Can you work these out from the model? Positions are in its coordinate system, mm. Face numbers are marked on the shaded views. A direction names the side the tool comes from. Round coordinates to 2 decimals unless told otherwise and drop trailing zeros. Loops run counter-clockwise (first coordinate to the right, second up) from the corner with the lowest first, then second, coordinate; pieces in that order, holes last. Notation, with made-up numbers: M 37.5,45.25 L 68.5,45.25 A29 ccw 68.5,80.25 Z; hole C 52,84.25 d1. An arc over 180 degrees is marked long. Return JSON: item names as keys, results as strings.
```python
from build123d import *

# Parameters (mm, degrees)
SM_BASE_FLANGE_2_DEPTH = 28
SKETCH_10_R            = 1.45
SKETCH_10_R_2          = 1.7
CUT_EXTRUDE_1_DEPTH    = 73.725511342
SKETCH_12_R            = 1.6
SKETCH_12_R_2          = 1.7
CUT_EXTRUDE_3_DEPTH    = 4


# Sheet-metal steps are written as plain solids
with BuildPart() as part:
    # 草图1 → 基体-法兰2 (new body)
    with BuildSketch(Plane.XY):
        with BuildLine():
            Line((-27.5, -25), (-27.5, 23))
            ThreePointArc((-27.5, 23), (-26.914213562, 24.414213562), (-25.5, 25))
            Line((-25.5, 25), (25.5, 25))
            ThreePointArc((25.5, 25), (26.914213562, 24.414213562), (27.5, 23))
            Line((27.5, 23), (27.5, -25))
            Line((27.5, -25), (30.5, -25))
            Line((30.5, -25), (30.5, 23))
            ThreePointArc((30.5, 23), (29.035533906, 26.535533906), (25.5, 28))
            Line((25.5, 28), (-25.5, 28))
            ThreePointArc((-25.5, 28), (-29.035533906, 26.535533906), (-30.5, 23))
            Line((-30.5, 23), (-30.5, -25))
            Line((-30.5, -25), (-27.5, -25))
        make_face()
    extrude(amount=SM_BASE_FLANGE_2_DEPTH)

    # 草图10 → 切除-拉伸1 (cut, through all)
    with BuildSketch(Plane.ZY.offset(30.5)):
        with Locations(Location((7, -15, 0), (0, 0, 270))):
            Circle(SKETCH_10_R)
        with Locations(Location((14, -15, 0), (0, 0, 270))):
            Circle(SKETCH_10_R_2)
        with Locations(Location((21, -15, 0), (0, 0, 270))):
            Circle(SKETCH_10_R)
        with Locations(Location((14, -8, 0), (0, 0, 270))):
            Circle(SKETCH_10_R)
        with Locations(Location((14, -22, 0), (0, 0, 270))):
            Circle(SKETCH_10_R)
        with BuildLine():
            Line((0, -25), (14, -25))
            ThreePointArc((14, -25), (5.397674733, -22.243255374), (0, -15))
            Line((0, -15), (0, -25))
        make_face()
        with BuildLine():
            ThreePointArc((28, -15), (22.602325267, -22.243255374), (14, -25))
            Line((14, -25), (28, -25))
            Line((28, -25), (28, -15))
        make_face()
    extrude(amount=-CUT_EXTRUDE_1_DEPTH, mode=Mode.SUBTRACT)

    # 草图12 → 切除-拉伸3 (cut)
    with BuildSketch(Plane(origin=(0, 28, 0), x_dir=(1, 0, 0), z_dir=(0, 1, 0))):
        with Locations(Location((-7, -14, 0), (0, 0, 270))):
            Circle(SKETCH_12_R)
        with Locations(Location((0, -7, 0), (0, 0, 270))):
            Circle(SKETCH_12_R)
        with Locations(Location((7, -14, 0), (0, 0, 270))):
            Circle(SKETCH_12_R)
        with Locations(Location((0, -14, 0), (0, 0, 270))):
            Circle(SKETCH_12_R_2)
        with Locations(Location((0, -21, 0), (0, 0, 270))):
            Circle(SKETCH_12_R)
    extrude(amount=-CUT_EXTRUDE_3_DEPTH, mode=Mode.SUBTRACT)


solid = part.part
```
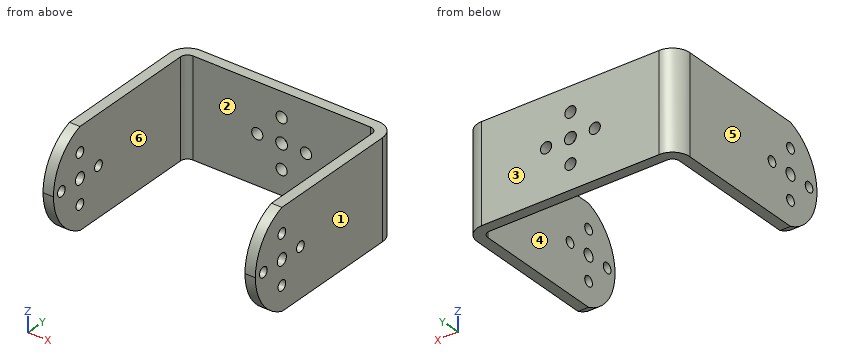
Q1. I'm going to push a flat-ended pin straight in: pin 1 Ø3 at (x, z) = (-1.5, 3) entering from -Y. Where does the tip first touch, or does it pass through?
Results:
{"pin 1": "stops at y = 25"}
Q2. Suppose I cut it at C-C, the plane x = 7. Please give me the cut outline in (y, z), plus the area to 3 significant figures.
Results:
{"outline": "M 25,0 L 28,0 L 28,12.4 L 25,12.4 Z; M 25,15.6 L 28,15.6 L 28,28 L 25,28 Z", "area": "74.4 mm2"}
Q3. Suppose I cut it at B-B, the plane y = 3. Please give me the cut outline in (x, z).
Results:
{"outline": "M -30.5,0 L -27.5,0 L -27.5,28 L -30.5,28 Z; M 27.5,0 L 30.5,0 L 30.5,28 L 27.5,28 Z"}
Q4. Suppose I cut it at A-A, the plane y = -8. Please give me the cut outline in (x, z).
Results:
{"outline": "M -30.5,0 L -27.5,0 L -27.5,12.55 L -30.5,12.55 Z; M -30.5,15.45 L -27.5,15.45 L -27.5,28 L -30.5,28 Z; M 27.5,0 L 30.5,0 L 30.5,12.55 L 27.5,12.55 Z; M 27.5,15.45 L 30.5,15.45 L 30.5,28 L 27.5,28 Z"}
Q5. If I drill on line 1 along Z through (x, y) = (-28, -15); line 2 along X through (y, z) = (26, 14); line 3 along X through (y, z) = (5.5, 25), over which ranges is the centre line in solid material (lowest first)?
Results:
{"line 1": "z = 0 to 5.55, 8.45 to 12.3, 15.7 to 19.55, 22.45 to 28", "line 2": "x = -29.5 to -8.6, -5.4 to -1.7, 1.7 to 5.4, 8.6 to 29.5", "line 3": "x = -30.5 to -27.5, 27.5 to 30.5"}
Q6. On a 3-axis mill with a long thin cutter (end or side, diameter ignored), from which of +Z, -Z, +X, -X, +Y, -Y can I reach the whole of each face in a straight line? I mean the marked faces 5 and 6. Say none if no direction works.
Results:
{"face 5": "+Z, -Z, -X, +Y, -Y", "face 6": "+Z, -Z, -Y"}
Q7. Suppose I cut it at D-D, the plane x = 0. Please give me the cut outline in (y, z).
Results:
{"outline": "M 25,0 L 28,0 L 28,5.4 L 25,5.4 Z; M 25,8.6 L 28,8.6 L 28,12.3 L 25,12.3 Z; M 25,15.7 L 28,15.7 L 28,19.4 L 25,19.4 Z; M 25,22.6 L 28,22.6 L 28,28 L 25,28 Z"}
Q8. Thinking about a two-plate mould opening in X: for the marked faces 1, 2, 3 and 4, which applies, pulls with the +X half, pulls with the -X half, needs draft (parallel to the pull), parting line crosses it, or undercut?
Results:
{"face 1": "pulls with the +X half", "face 2": "undercut", "face 3": "needs draft", "face 4": "undercut"}
